```python
from build123d import *

# Parameters (mm, degrees)
PAD_DEPTH       = 15
SKETCH003_R     = 6
PAD001_DEPTH    = 1
SKETCH005_R     = 3.9
PAD002_DEPTH    = 1
SKETCH004_R     = 6
PAD003_DEPTH    = 1
SKETCH_R        = 3.9
PAD004_DEPTH    = 1
POCKET_DEPTH    = 15.001
SKETCH012_W     = 29
SKETCH012_H     = 8.6
SKETCH012_W_2   = 26
SKETCH012_H_2   = 2.6
PAD005_DEPTH    = 11
SKETCH013_W     = 26
SKETCH013_H     = 2.6
POCKET001_DEPTH = 21.471
PAD006_DEPTH    = 2.6
POCKET002_DEPTH = 38.3479098694
FILLET_R        = 7.499
POCKET003_DEPTH = 8.601
CHAMFER_SIZE    = 1
CHAMFER001_SIZE = 1
CHAMFER002_SIZE = 0.59


with BuildPart() as part:
    # Sketch001 → Pad (new body)
    with BuildSketch(Plane.XY):
        with BuildLine():
            ThreePointArc((34.031969, 3.1), (29.481969, -1.45), (34.031969, -6))
            Line((34.031969, -6), (64.031969, -6))
            Line((64.031969, -6), (64.031969, -10))
            Line((34.3372726559, -10), (64.031969, -10))
            Line((29, -21.4458181471), (34.3372726559, -10))
            Line((29, -30.8675547205), (29, -21.4458181471))
            Line((0, -30.8675547205), (29, -30.8675547205))
            Line((0, -20.178085), (0, -30.8675547205))
            Line((0, -20.178085), (27.278085, 7.1))
            Line((27.278085, 7.1), (64.031969, 7.1))
            Line((64.031969, 7.1), (64.031969, 3.1))
            Line((34.031969, 3.1), (64.031969, 3.1))
        make_face()
    extrude(amount=PAD_DEPTH)

    # Sketch003 → Pad001 (join)
    with BuildSketch(Plane.XZ.offset(-3.1)):
        with Locations((57, 7.5)):
            Circle(SKETCH003_R)
    extrude(amount=PAD001_DEPTH)

    # Sketch005 (on Face16 of Pad001) → Pad002 (join)
    with BuildSketch(Plane.XZ.offset(-2.1)):
        with Locations((57, 7.5)):
            Circle(SKETCH005_R)
    extrude(amount=PAD002_DEPTH)

    # Sketch004 → Pad003 (join)
    with BuildSketch(Plane(origin=(0, -6, 0), x_dir=(-1, 0, 0), z_dir=(0, 1, 0))):
        with Locations((-57, 7.5)):
            Circle(SKETCH004_R)
    extrude(amount=PAD003_DEPTH)

    # Sketch → Pad004 (join)
    with BuildSketch(Plane(origin=(0, -5, 0), x_dir=(-1, 0, 0), z_dir=(0, 1, 0))):
        with Locations((-57, 7.5)):
            Circle(SKETCH_R)
    extrude(amount=PAD004_DEPTH)

    # Sketch008 → Pocket (cut, through all)
    with BuildSketch(Plane.XY):
        with BuildLine():
            ThreePointArc((13.0697507591, -14.0345267419), (12.559643278, -16.2651404862), (14.5155135985, -17.4527509473))
            Line((14.5155135985, -17.4527509473), (25.1710077735, -16.6064336644))
            ThreePointArc((25.1710077735, -16.6064336644), (25.7569811778, -16.3971334306), (26.15789695, -15.9212784504))
            Line((26.15789695, -15.9212784504), (28.5635079634, -10.7624289841))
            ThreePointArc((28.5635079634, -10.7624289841), (28.6753075146, -9.9775618701), (28.3317651199, -9.2630731374))
            Line((28.3317651199, -9.2630731374), (24.7051920017, -5.3153901784))
            ThreePointArc((24.7051920017, -5.3153901784), (23.3062813222, -4.6824374231), (21.8808496163, -5.2531604134))
            Line((13.0697507591, -14.0345267419), (21.8808496163, -5.2531604134))
        make_face()
    extrude(amount=POCKET_DEPTH, mode=Mode.SUBTRACT)

    # Sketch012 (on Face4 of Pocket) → Pad005 (join)
    with BuildSketch(Plane(origin=(0, 0, 0), x_dir=(1, 0, 0), z_dir=(0, 0, -1))):
        with Locations((14.5, 26.5675547205)):
            Rectangle(SKETCH012_W, SKETCH012_H)
        with Locations((14.159, 26.5675547205)):
            Rectangle(SKETCH012_W_2, SKETCH012_H_2, mode=Mode.SUBTRACT)
    extrude(amount=PAD005_DEPTH)

    # Sketch013 (on Face30 of Pad005) → Pocket001 (cut)
    with BuildSketch(Plane(origin=(0, 0, -11), x_dir=(1, 0, 0), z_dir=(0, 0, -1))):
        with Locations((14.159, 26.5675547205)):
            Rectangle(SKETCH013_W, SKETCH013_H)
    extrude(amount=-POCKET001_DEPTH, mode=Mode.SUBTRACT)

    # Sketch014 (on Face36 of Pocket001) → Pad006 (join)
    with BuildSketch(Plane.XZ.offset(25.2675547205)):
        Polygon((27.159, -0.9), (27.159, 10.471), (17.1566665969, 10.471), align=None)
    extrude(amount=PAD006_DEPTH)

    # Sketch015 (on Face15 of Pad006) → Pocket002 (cut, through all)
    with BuildSketch(Plane(origin=(32.0346452503, -14.9380004065, 0), x_dir=(0.4226182617, 0.906307787, 0), z_dir=(0.906307787, -0.4226182617, 0))):
        Polygon((-5.6805823956, 10.8894220066), (-2.8269007902, 7.5), (-5.6805823956, 4.1105779934), align=None)
        Polygon((-3.9568261963, 13.5), (-0.8660508916, 9.828973136), (2.224724413, 13.5), align=None)
        Polygon((3.9484806124, 10.8894220066), (1.0947990069, 7.5), (3.9484806124, 4.1105779934), align=None)
        Polygon((-0.8660508916, 5.171026864), (2.224724413, 1.5), (-3.9568261963, 1.5), align=None)
    extrude(amount=-POCKET002_DEPTH, mode=Mode.SUBTRACT)

    # Fillet
    fillet_edges = [part.edges().sort_by_distance(p)[0] for p in [
        (64.031969, -8, 15),
        (64.031969, -8, 0),
        (64.031969, 5.1, 0),
        (64.031969, 5.1, 15),
    ]]
    fillet(fillet_edges, radius=FILLET_R)

    # Sketch016 (on Face15 of Fillet) → Pocket003 (cut, through all)
    with BuildSketch(Plane(origin=(0, -22.2675547205, 0), x_dir=(-1, 0, 0), z_dir=(0, 1, 0))):
        with BuildLine():
            Line((-10.199, -11), (-10.199, -5))
            ThreePointArc((-10.199, -5), (-14.199, -1.0000000634), (-18.199, -5))
            Line((-18.199, -11), (-18.199, -5))
            Line((-10.199, -11), (-18.199, -11))
        make_face()
    extrude(amount=-POCKET003_DEPTH, mode=Mode.SUBTRACT)

    # Chamfer
    chamfer_edges = [part.edges().sort_by_distance(p)[0] for p in [
        (17.4753, -9.643844, 15),
        (26.518479, -7.289232, 0),
    ]]
    chamfer(chamfer_edges, length=CHAMFER_SIZE)

    # Chamfer001
    chamfer001_edges = [part.edges().sort_by_distance(p)[0] for p in [
        (13.639043, -6.539043, 0),
        (41.905527, 7.1, 0),
        (45.435121, -10, 0),
        (45.435121, -10, 15),
        (29.481969, -1.45, 0),
        (29.481969, -1.45, 15),
        (41.905527, 7.1, 15),
        (13.639043, -6.539043, 15),
        (27.278085, 7.1, 7.5),
        (0, -20.178085, 7.5),
        (31.668636, -15.722909, 15),
        (29, -26.156686, 15),
        (0, -25.52282, 15),
        (14.5, -30.867555, 15),
        (29, -30.867555, 7.5),
        (0, -30.867555, 7.5),
        (29, -22.267555, -5.5),
        (29, -30.867555, -5.5),
        (31.668636, -15.722909, 0),
    ]]
    chamfer(chamfer001_edges, length=CHAMFER001_SIZE)

    # Chamfer002
    chamfer002_edges = [part.edges().sort_by_distance(p)[0] for p in [
        (29, -21.856686, 0),
    ]]
    chamfer(chamfer002_edges, length=CHAMFER002_SIZE)


solid = part.part
```
The listing builds one solid part. Answer for the finished solid, in the listing's coordinates (mm). A direction names the side the tool comes from. Coordinates: 2 decimals unless noted, no trailing zeros. Loops run counter-clockwise (first coordinate to the right, second up) from the corner with the lowest first, then second, coordinate; pieces in that order, holes last. Notation, with made-up numbers: (0.25, 59) - (52.25, 59) arc R29 cw to (52.25, 84) - close; hole circle Ø2 at (78.25, 44.25). An arc over 180 degrees is marked (long way). Use a Markdown table: item, result. Add a question column.
1) For faces 1 (the flat face through (10.199, -29, -8)), 2 (the flat face through (19.14, -4.57, 7.45)), 3 (the flat face through (11, -22.268, -2)), 4 (the cylindrical face through (29.483, -1.35, 7.409)), 5 (the conical face through (23.29, -4.3, 14.38)), determine the directions among +Z, -Z, +X, -X, +Y, -Y from which every point of the face is accessible in a straight line to the end or side of a thin tool.
2) The part is cut by section C-C, the plane y = -26. Give the vertices of the cut face in (x, z).
3) The part is cut by section A-A, the plane x = 38. Give the vertices of the cut face in (y, z), and give its area (3 significant figures).
4) The part is cut by section D-D, the plane y = -1.45. Give the vertices of the cut face in (x, z), and give its area (3 significant figures).
5) Given pin 1 (3.5 mm diameter, centred on x = 16.5, y = -8.5, fed in from -Z); pin 2 (1 mm diameter, centred on y = -15.5, z = 0, fed in from -X); pin 3 (3 mm diameter, centred on y = -25.5, z = 3, fed in from +X); pin 4 (10 mm diameter, centred on x = 37.5, y = -16, fed in from +Z), each flat-ended and moving along its own axis, determine where each tip first touches the part or whether it passes through.
6) The part is cut by section B-B, the plane z = -7. Give the vertices of the cut face in (x, y), and give its area (3 significant figures).
7) Find the intervals of material crossed by line 1 (Y direction, x = 4, z = -2.75); line 2 (Y direction, x = 53, z = 14); line 3 (Z direction, x = 15.5, y = -7.5), in increasing order.
8) The mould has two halves that part along Y. Classify faces 6 (the conical face through (61.199, 6.926, 2.729)), 7 (the flat face through (10.199, -24, -8)), 8 (the flat face through (1.159, -27, 0)): released by +Y, released by -Y, zero draft, split by the parting line, or undercut.
Here are the results:
| question | item | result |
|---|---|---|
| 1 | face 1 | -Z, +Y, -Y |
| 1 | face 2 | none |
| 1 | face 3 | -Z, +X, -X, +Y |
| 1 | face 4 | +Z, -Z |
| 1 | face 5 | +Z |
| 2 | outline | (0, -11) - (1.16, -11) - (1.16, 10.47) - (17.16, 10.47) - (27.16, -0.9) - (27.16, -11) - (29, -11) - (29, 14) - (28, 15) - (1, 15) - (0, 14) - close |
| 3 | outline | (-10, 1) - (-9, 0) - (-7, 0) - (-6, 1) - (-6, 14) - (-7, 15) - (-9, 15) - (-10, 14) - close; (3.1, 1) - (4.1, 0) - (6.1, 0) - (7.1, 1) - (7.1, 14) - (6.1, 15) - (4.1, 15) - (3.1, 14) - close |
| 3 | area | 116 mm^2 |
| 4 | outline | (18.73, 1) - (20.14, 0) - (28.48, 0) - (29.48, 1) - (29.48, 14) - (28.48, 15) - (20.14, 15) - (18.73, 14) - close |
| 4 | area | 159 mm^2 |
| 5 | pin 1 | stops at z = 0 |
| 5 | pin 2 | stops at x = 5.23 |
| 5 | pin 3 | stops at x = 29 |
| 5 | pin 4 | passes through |
| 6 | outline | (0, -29.87) - (1, -30.87) - (10.2, -30.87) - (10.2, -27.87) - (1.16, -27.87) - (1.16, -25.27) - (10.2, -25.27) - (10.2, -22.27) - (0, -22.27) - close; (18.2, -30.87) - (28, -30.87) - (29, -29.87) - (29, -23.27) - (28, -22.27) - (18.2, -22.27) - (18.2, -25.27) - (27.16, -25.27) - (27.16, -27.87) - (18.2, -27.87) - close |
| 6 | area | 132 mm^2 |
| 7 | line 1 | y = -30.87 to -27.87, -25.27 to -22.27 |
| 7 | line 2 | y = -10 to -6, 3.1 to 7.1 |
| 7 | line 3 | z = 0 to 1.5, 4.44 to 10.56, 13.5 to 15 |
| 8 | face 6 | released by +Y |
| 8 | face 7 | zero draft |
| 8 | face 8 | undercut |
